Autodesk Fusion 360 part; units mm, degrees
sketch "Base" plane through (0, 0, 0) normal (0, 0, 1) x (1, 0, 0) in component "UltrasonicSensorSuport"
  line L0 (18, 10.5) -> (-18, 10.5)
  line L1 (-18, 10.5) -> (-18, -10.5)
  line L2 (-18, -10.5) -> (18, -10.5)
  line L3 (18, -10.5) -> (18, 10.5)
  line L4 (18, 10.5) -> (-18, -10.5) construction
  line L5 (-18, 10.5) -> (18, -10.5) construction
  line L6 (-20, 12.5) -> (-20, -12.5)
  line L7 (-20, -12.5) -> (20, -12.5)
  line L8 (20, -12.5) -> (20, 12.5)
  line L9 (20, 12.5) -> (-20, 12.5)
  line L10 (-24, -16.5) -> (24, -16.5)
  line L11 (24, -16.5) -> (24, 16.5)
  line L12 (24, 16.5) -> (-24, 16.5)
  line L13 (-24, 16.5) -> (-24, -16.5)
  circle A0 centre (-16.4, 8.9) radius 1.55
  line L14 (0, 0) -> (-18, 0) construction
  line L15 (0, 0) -> (0, 10.5) construction
  circle A1 centre (-16.4, -8.9) radius 1.55
  circle A2 centre (16.4, 8.9) radius 1.55
  circle A3 centre (16.4, -8.9) radius 1.55
  line L16 (0, 10.5) -> (0, 12.5) construction
  line L17 (0, 12.5) -> (-5.5, 12.5) construction
  line L18 (-5.5, 7.5) -> (5.5, 7.5)
  line L19 (5.5, 7.5) -> (5.5, 19.5)
  line L20 (-5.5, 7.5) -> (-5.5, 19.5)
  line L21 (-5.5, 19.5) -> (5.5, 19.5)
  line L22 (0, 7.5) -> (0, 0) construction
  line L23 (5.5, 7.5) -> (8.5, 7.5) construction
  line L24 (8.5, 7.5) -> (8.5, 10.5) construction
  point P0 (0, 10.5)
  dimension "d8" = 36
  dimension "d9" = 21
  dimension "d12" = 2
  dimension "d13" = 6
  dimension "d46" = 3.1
  dimension "d47" = 1.6
  dimension "d48" = 1.6
  dimension "d52" = 11
  dimension "d53" = 12
  dimension "d54" = 3
  dimension "d55" = 3
extrude "Extrude1" add sketch "Base" along normal blind 3 contours L0 L1 L2 L3 L18 L19 L20 | L0 L1 L2 L3 L6 L7 L8 L9 L19 L20 | L0 L18 L19 L20 | L0 L9 L19 L20 | L6 L7 L8 L9 L10 L11 L12 L13 L19 L20 | L9 L12 L19 L20 | A0 | A1 | A2 | A3 makes body 1 in component "UltrasonicSensorSuport"
sketch "BaseExtension" plane through (0, 0, 3) normal (0, 0, 1) x (-1, 0, 0) in component "UltrasonicSensorSuport"
  line L0 (24, -16.5) -> (24, 16.5)
  line L1 (24, 16.5) -> (-24, 16.5)
  line L2 (-24, 16.5) -> (-24, -16.5)
  line L3 (-24, -16.5) -> (24, -16.5)
  line L4 (20, 12.5) -> (-20, 12.5)
  line L5 (-20, 12.5) -> (-20, -12.5)
  line L6 (-20, -12.5) -> (20, -12.5)
  line L7 (20, -12.5) -> (20, 12.5)
  circle A0 centre (-20.35, 12.85) radius 1.55
  circle A1 centre (20.35, -12.85) radius 1.55
  point P0 (-24, -16.5)
  point P1 (24, -16.5)
  point P2 (24, 16.5)
  point P3 (-24, 16.5)
  dimension "d16" = -4
  dimension "d19" = 3.1
  dimension "d20" = 3.1
  dimension "d21" = 3.65
  dimension "d22" = 3.65
  dimension "d23" = 3.65
  dimension "d24" = 3.65
extrude "Extrude2" add sketch "BaseExtension" along normal blind 6.5 separate body contours L4 L5 L6 L7 A0 A1 | L4 L5 A0 | L6 L7 A1 picked at (-19.557, 11.9554) picked at (20.9471, -13.4767) makes body 2 at (7.0018, 4.0327, 3) in component "UltrasonicSensorSuport"
shell "Shell1" thickness 2 removed faces 1 at (-8, 5.5, 0) on bodies 1 in component "UltrasonicSensorSuport"
sketch "TransducerHoles" plane through (0, 0, 9.5) normal (0, 0, 1) x (-1, 0, 0) in component "UltrasonicSensorSuport"
  line L0 (20, -12.5) -> (20, 12.5)
  line L1 (20, 12.5) -> (-20, 12.5)
  line L2 (-20, 12.5) -> (-20, -12.5)
  line L3 (-20, -12.5) -> (20, -12.5)
  circle A0 centre (-9.5, 0) radius 9
  circle A1 centre (9.5, 0) radius 9
  line L4 (20, -12.5) -> (20, 12.5)
  line L5 (-20, 12.5) -> (-20, -12.5)
  line L6 (20, 0) -> (-20, 0) construction
  line L7 (24, -16.5) -> (24, 16.5)
  line L8 (-24, -16.5) -> (24, -16.5)
  line L9 (24, 16.5) -> (-24, 16.5)
  line L10 (-24, 16.5) -> (-24, -16.5)
  line L11 (-20, -12.5) -> (20, -12.5)
  line L12 (20, 12.5) -> (-20, 12.5)
  line L13 (0, -12.5) -> (0, 12.5) construction
  line L14 (9.5, 0) -> (0, 0) construction
  line L15 (0, 0) -> (-9.5, 0) construction
  line L16 (9.5, -9) -> (-9.5, -9)
  line L17 (9.5, 9) -> (-9.5, 9)
  dimension "d33" = 18
  dimension "d34" = 18
  dimension "d35" = 19
extrude "Extrude7" cut sketch "TransducerHoles" against normal up to surface (9.5 mm away) contours A0 | A0 A1 L16 L17 | A1 bodies 1 2 in component "UltrasonicSensorSuport"
extrude "Extrude8" add 1 faces at (-3.1667, 14, 3) along direction (0, 0, 1) blind 2 on bodies 1 bodies 1 2 in component "UltrasonicSensorSuport"
extrude "Extrude9" cut sketch "Base" along normal up to surface (9.5 mm away) contours A0 | A3 bodies 1 in component "UltrasonicSensorSuport"
extrude "Extrude11" add 1 faces at (7.3333, -15.8333, 0) along direction (0, 0, -1) blind 21 on bodies 1 bodies 1 in component "UltrasonicSensorSuport"
extrude "Extrude10" cut sketch "Base" along normal blind 2 contours L0 L18 L19 L20 | L0 L9 L19 L20 | L9 L12 L19 L20 | L12 L19 L20 L21 bodies 1 in component "UltrasonicSensorSuport"
extrude "Extrude14" cut 1 faces at (-1.8333, 15.1667, 0) along direction (0, 0, -1) up to surface (21 mm away) on bodies 1 bodies 1 in component "UltrasonicSensorSuport"
extrude "Extrude16" cut 1 faces at (-5.5, 15.8333, -6) along direction (-1, 0, 0) blind 2 on bodies 1 bodies 1 in component "UltrasonicSensorSuport"
extrude "Extrude17" cut 1 faces at (5.5, 15.8333, -6) along direction (1, 0, 0) blind 2 on bodies 1 bodies 1 in component "UltrasonicSensorSuport"
sketch "MountingScrewHole" plane through (24, 0, 0) normal (1, 0, 0) x (0, 1, 0) in component "UltrasonicSensorSuport"
  line L0 (16.5, -21) -> (16.5, 5)
  line L1 (16.5, 5) -> (-16.5, 5)
  line L2 (-16.5, 5) -> (-16.5, -21)
  line L3 (16.5, 5) -> (-16.5, -21) construction
  line L4 (16.5, -21) -> (-16.5, 5) construction
  circle A0 centre (0, -8) radius 1.55
  line L5 (-16.5, -21) -> (16.5, -21)
  point P0 (0, -8)
  dimension "d63" = 3.1
extrude "Extrude13" cut sketch "MountingScrewHole" against normal up to surface (2 mm away) contours A0 bodies 1 in component "UltrasonicSensorSuport"
ref_plane "WorkPlane1" through (0, 0, -8) normal (1, 0, 0) x (0, 1, 0) in component "UltrasonicSensorSuport"
mirror "Mirror1" about plane through (0, 0, -8) normal (1, 0, 0) of "Extrude13" in component "UltrasonicSensorSuport"
pattern_linear "00000000-0000-0000-0000-000000000000" [suppressed]
component "UltrasonicSensorSuport" placed x (1, 0, 0) y (0, 1, 0) z (0, 0, 1) at (0, 0, 0)
equation "M3 = 3 mm"
equation "Length = 3.6 cm"
equation "Width = 2.1 cm"
equation "Height = 1 mm"
equation "TransducerHeight = 1.3 cm"
equation "TransducerDiameter = 1.6 cm"
equation "TransducersCenterDistance = 3.5 cm - TransducerDiameter"
equation "d8 = Length"
equation "d9 = Width"
equation "PrintMargin = 2 mm"
equation "BaseThickness = 3 mm"
equation "d12 = PrintMargin"
equation "d13 = PrintMargin + BaseThickness + 1 mm"
equation "d14 = BaseThickness"
equation "d16 = -PrintMargin - 2 mm"
equation "d17 = TransducerHeight / 2"
equation "d19 = M3 + 0.1 mm"
equation "d20 = d19"
equation "d21 = M3 / 2 + 0.15 mm + 2 mm"
equation "d22 = M3 / 2 + 0.15 mm + 2 mm"
equation "d23 = d22"
equation "d24 = d21"
equation "d33 = TransducerDiameter + PrintMargin"
equation "d34 = d33"
equation "d35 = TransducersCenterDistance"
equation "d37 = PrintMargin"
equation "d40 = PrintMargin"
equation "d46 = M3 + 0.1 mm"
equation "d47 = 0.1 mm + M3 / 2"
equation "d48 = d47"
equation "d63 = M3 + 0.1 mm"

Autodesk Fusion 360 part; units mm, degrees
sketch "Front" plane through (0, 0, 0) normal (0, 1, 0) x (1, 0, 0)
  line L0 (23.5, -23.5) -> (-23.5, -23.5)
  line L1 (-23.5, -23.5) -> (-23.5, 23.5)
  line L2 (-23.5, 23.5) -> (23.5, 23.5)
  line L3 (23.5, 23.5) -> (23.5, -23.5)
  line L4 (23.5, -23.5) -> (-23.5, 23.5) construction
  line L5 (-23.5, -23.5) -> (23.5, 23.5) construction
  line L6 (-26.5, 26.5) -> (26.5, 26.5)
  line L7 (26.5, 26.5) -> (26.5, -26.5)
  line L8 (26.5, -26.5) -> (-26.5, -26.5)
  line L9 (-26.5, -26.5) -> (-26.5, 26.5)
  circle A0 centre (3.9904, -6.933) radius 8
  circle A1 centre (0, -15) radius 2.5
  circle A2 centre (12.9904, -7.5) radius 2.5
  circle A3 centre (12.9904, 7.5) radius 2.5
  circle A4 centre (0, 15) radius 2.5
  circle A5 centre (-12.9904, 7.5) radius 2.5
  circle A6 centre (-12.9904, -7.5) radius 2.5
  line L10 (0, 0) -> (0, -23.5) construction
  line L11 (-23.5, 0) -> (23.5, 0)
  circle A7 centre (3.9904, 6.933) radius 8
  dimension "d13" = 47
  dimension "d14" = 47
  dimension "d23" = 16
  dimension "d26" = 5
  dimension "d27" = 15
  dimension "d29" = 360
  dimension "d53" = 9
  dimension "d54" = 9
extrude "Extrude4" add sketch "Front" along normal blind 3 contours L0 L1 L3 A0 A1 A2 L11 | L1 L2 L3 A3 A4 L11 A7 | A0 L11 | L11 A7 | A0 A1 A2 A7 | A0 A3 A4 A7 | A0 A2 | A0 A2 | A3 A7 | A3 A7 | A0 A1 | A0 A1 | A4 A7 | A4 A7 | A5 | A6 makes body 1
extrude "Extrude5" add sketch "Front" along normal blind 60 contours L6 L7 L8 L9 bodies 1
extrude "Extrude6" cut sketch "Front" along normal up to surface (3 mm away) contours A0 L11 | L11 A7 | A0 A3 A4 A7 | A3 A7 | A4 A7 picked at (13.1407, 7.417) picked at (0.1211, 13.399) bodies 1
extrude "Extrude7" cut sketch "Front" along normal up to surface (3 mm away) contours A0 A2 | A0 A2 | A3 A7 | A3 A7 | A0 A1 | A0 A1 | A4 A7 | A4 A7 | A5 | A6 bodies 1
sketch "BottomHole" plane through (0, 0, -26.5) normal (0, 0, -1) x (1, 0, 0)
  line L0 (26.5, 0) -> (-26.5, 0)
  line L1 (-26.5, 0) -> (-26.5, -60)
  line L2 (-26.5, -60) -> (26.5, -60)
  line L3 (26.5, -60) -> (26.5, 0)
  line L4 (-23.5, -3) -> (23.5, -3)
  line L5 (23.5, -3) -> (23.5, -60)
  line L6 (23.5, -60) -> (-23.5, -60)
  line L7 (-23.5, -60) -> (-23.5, -3)
  line L8 (23.5, -3) -> (23.5, -33)
  line L9 (23.5, -33) -> (0, -25.5905)
  line L10 (0, -25.5905) -> (-23.5, -33)
  line L11 (-23.5, -33) -> (23.5, -33)
  line L12 (16.4289, -3) -> (23.5, -10.0711)
  line L13 (0, -3) -> (0, -25.5905)
  line L14 (-16.4289, -3) -> (-23.5, -10.0711)
  dimension "d55" = 30
  dimension "d57" = 145
  dimension "d60" = 45
  dimension "d61" = 5
fillet "Fillet1" radius 2 6 edges at (26.5, 30, 26.5) (-26.5, 30, 26.5) (-26.5, 30, -26.5) (26.5, 30, -26.5) (0, 60, -26.5) (0, 60, 26.5) on bodies 1
fillet "Fillet2" radius 2 8 edges at (-25.9142, 0, 25.9142) (-26.5, 0, 0) (-25.9142, 0, -25.9142) (0, 0, -26.5) (25.9142, 0, -25.9142) (26.5, 0, 0) (25.9142, 0, 25.9142) (0, 0, 26.5) on bodies 1
sketch "Mounting" plane through (-26.5, 0, 0) normal (-1, 0, 0) x (0, -1, 0)
  line L0 (-2, -24.5) -> (-2, 24.5)
  line L1 (-2, 24.5) -> (-60, 24.5)
  line L2 (-60, 24.5) -> (-60, -24.5)
  line L3 (-60, -24.5) -> (-2, -24.5)
  line L4 (-60, 14.5) -> (-2, 14.5)
  line L5 (-2, 14.5) -> (-2, 10.5)
  line L6 (-2, 10.5) -> (-60, 10.5)
  line L7 (-60, 14.5) -> (-60, 10.5)
  dimension "d36" = 4
  dimension "d37" = 10
extrude "Extrude8" add sketch "Mounting" along normal blind 5 separate body contours L0 L2 L4 L5 L6 L7 makes body 2
sketch "ScrewHoles" plane through (0, 0, 14.5) normal (0, 0, 1) x (-1, 0, 0)
  line L0 (26.5, -60) -> (31.5, -60)
  line L1 (31.5, -60) -> (31.5, -2)
  line L2 (31.5, -2) -> (26.5, -2)
  line L3 (26.5, -2) -> (24.5, -2)
  line L4 (24.5, -2) -> (24.5, -58)
  line L5 (26.5, -60) -> (24.5, -58)
  line L6 (26.5, -60) -> (26.5, -2)
  circle A0 centre (29, -51) radius 1.6
  circle A1 centre (29, -31) radius 1.6
  circle A2 centre (29, -11) radius 1.6
  line L7 (26.5, -60) -> (31.5, -2) construction
  line L8 (31.5, -60) -> (26.5, -2) construction
  line L9 (26.5, -2) -> (26.5, -60)
  dimension "d40" = 3.2
  dimension "d43" = 0
  dimension "d44" = 20
extrude "Extrude9" cut sketch "ScrewHoles" against normal up to surface (4 mm away) contours A0 | A1 | A2 bodies 1
sketch "Sketch5" plane through (0, 60, 0) normal (0, 1, 0) x (-1, 0, 0)
  line L0 (23.5, -23.5) -> (-23.5, -23.5)
  line L1 (-23.5, -23.5) -> (-23.5, 23.5)
  line L2 (-23.5, 23.5) -> (23.5, 23.5)
  line L3 (23.5, 23.5) -> (23.5, -23.5)
  line L4 (-26.5, -24.5) -> (26.5, -24.5)
  line L5 (26.5, -24.5) -> (26.5, 24.5)
  line L6 (26.5, 24.5) -> (-26.5, 24.5)
  line L7 (-26.5, 24.5) -> (-26.5, -24.5)
  line L8 (26.5, 14.5) -> (31.5, 14.5)
  line L9 (26.5, -24.5) -> (26.5, 24.5)
  line L10 (26.5, 24.5) -> (31.5, 14.5)
extrude "Extrude10" add sketch "Sketch5" against normal blind 2.5 separate body contours L5 L8 L9 L10 makes body 3
ref_plane "WorkPlane1" through (-29, 31, 12.5) normal (0, 1, 0) x (0, 0, -1)
mirror "Mirror1" about plane through (-29, 31, 12.5) normal (0, 1, 0) of bodies 3 makes body 4
combine "Combine1" operation add target body 2 tool bodies 3 4
mirror "Mirror2" about plane through (0, 0, 0) normal (1, 0, 0) of bodies 2 makes body 5
combine "Combine2" operation add target body 1 tool bodies 5 2
equation "Diameter = 37 mm"
equation "Length = 50 mm"
equation "ShaftDiameter = 6 mm"
equation "ShaftLength = 15 mm"
equation "PrintThickness = 3 mm"
equation "d13 = Diameter + 10 mm"
equation "d14 = d13"
equation "d19 = PrintThickness"
equation "d21 = Length + 10 mm"
equation "d23 = ShaftDiameter + 10 mm"
The model under review builds one solid part; all positions refer to its coordinate system, in mm. A direction names the side the tool comes from. Round coordinates to 2 decimals unless told otherwise and drop trailing zeros. Write each loop counter-clockwise with the first axis right and the second up, starting at its lowest first coordinate (ties: lowest second). Pieces come first, ordered by that corner, then holes.
(1) Wall thickness on L1, parallel to Z at x = -16.5, y = 16; L2, parallel to Z at x = 0, y = 1.2: over which ranges is each line inside the solid? List them lowest first.
(2) We need section A-A on y = 45. Give the boundary of the cut face in (x, z).
(3) We need section B-B on x = -8.5. Give the boundary of the cut face in (y, z), and give its area (3 significant figures).
(4) We need section D-D on x = 9.5. Give the boundary of the cut face in (y, z), and give its area (3 significant figures).
(5) Mouldability with a two-part tool opening along X and no side actions: class faces 1 (the flat face through (29.035, 58.768, 19.43)), 2 (the flat face through (0, 31, 23.5)), 3 (the flat face through (29, 31, 10.5)) as +X half, -X half, draft (parallel to the pull), parting line (faces both ways), or undercut.
(6) Machinability: for faces 4 (the flat face through (-29, 31, 10.5)), 5 (the flat face through (28, 57.5, 17)), 6 (the flat face through (-28, 57.5, 17)), 7 (the cylindrical face through (7.93, 1.479, -13.896)), which of the approach directions +Z, -Z, +X, -X, +Y, -Y give a long, thin tool a straight path to every point of the face, cutting with its end or side? Answer none if there is none.
(7) Insertion check: pin 1 (4 mm diameter, centred on x = 0, z = -15, fed in from -Y); pin 2 (8 mm diameter, centred on y = 16.5, z = 16.5, fed in from -X); pin 3 (5.5 mm diameter, centred on x = -29.5, y = 20.5, fed in from +Z); pin 4 (4 mm diameter, centred on x = 29.5, z = 19.5, fed in from -Y). Each pin has a flat end and moves straight along its axis. Give the tip position at first contact, or say it passes through.
(8) We need section C-C on z = 7.5. Give the boundary of the cut face in (x, y), and give its area (3 significant figures).
Findings below:
1. L1: z = -26.5 to -23.5, 23.5 to 26.5
1. L2: z = -26.33 to -17.5, 0 to 12.5, 17.5 to 26.33
2. outline: (-31.5, 10.5) - (-26.5, 10.5) - (-26.5, -24.5) arc R2 ccw to (-24.5, -26.5) - (24.5, -26.5) arc R2 ccw to (26.5, -24.5) - (26.5, 10.5) - (31.5, 10.5) - (31.5, 14.5) - (26.5, 14.5) - (26.5, 24.5) arc R2 ccw to (24.5, 26.5) - (-24.5, 26.5) arc R2 ccw to (-26.5, 24.5) - (-26.5, 14.5) - (-31.5, 14.5) - close; hole (-23.5, -23.5) - (23.5, -23.5) - (23.5, 23.5) - (-23.5, 23.5) - close
3. outline: (0, -24.5) arc R2 ccw to (2, -26.5) - (58, -26.5) arc R2 ccw to (60, -24.5) - (60, -23.5) - (3, -23.5) - (3, 23.5) - (60, 23.5) - (60, 24.5) arc R2 ccw to (58, 26.5) - (2, 26.5) arc R2 ccw to (0, 24.5) - close
3. area: 498 mm2
4. outline: (0, -24.5) arc R2 ccw to (2, -26.5) - (58, -26.5) arc R2 ccw to (60, -24.5) - (60, -23.5) - (3, -23.5) - (3, -12.73) - (0, -12.73) - close; (0, -1.13) - (3, -1.13) - (3, 23.5) - (60, 23.5) - (60, 24.5) arc R2 ccw to (58, 26.5) - (2, 26.5) arc R2 ccw to (0, 24.5) - close
4. area: 463 mm2
5. face 1: +X half
5. face 2: undercut
5. face 3: draft
6. face 4: -Z, -X, +Y, -Y
6. face 5: +Z, +X
6. face 6: +Z, -X
6. face 7: +Y, -Y
7. pin 1: passes through
7. pin 2: stops at x = -31.5
7. pin 3: stops at z = 14.5
7. pin 4: stops at y = 2
8. outline: (-26.5, 2) arc R2 ccw to (-24.5, 0) - (-15.49, 0) - (-15.49, 3) - (-23.5, 3) - (-23.5, 60) - (-26.5, 60) - close; (-10.49, 0) - (10.49, 0) - (10.49, 3) - (-10.49, 3) - close; (15.49, 0) - (24.5, 0) arc R2 ccw to (26.5, 2) - (26.5, 60) - (23.5, 60) - (23.5, 3) - (15.49, 3) - close
8. area: 469 mm2
